Could you check a few things on this model? Use its own coordinates, in mm. A direction names the side the tool comes from. Give positions to 0.01 mm unless a question says otherwise; leave off trailing zeros. Write each loop counter-clockwise with the first axis right and the second up, starting at its lowest first coordinate (ties: lowest second). Pieces come first, ordered by that corner, then holes. Notation, with made-up numbers: M -31.5,73.25 L 7.5,73.25 A28 ccw 7.5,105.25 Z; hole C 5.25,28.5 d10. An arc over 180 degrees is marked long. Use one line per item in the form item = value.
from build123d import *

# Parameters (mm, degrees)
F0_W      = 76.2
F0_H      = 38.1
F1_DEPTH  = 17.78
F2_R      = 6.35
F3_DEPTH  = 15.24
F5_DEPTH  = 5.332479
F6_DEPTH  = 5.837152
F7_R      = 1.27
F8_DEPTH  = 67.31
F9_R      = 5.08
F10_R     = 5.08
F11_W     = 13.054326
F11_H     = 13.088878
F12_DEPTH = 7.62
F13_W     = 11.43
F13_H     = 11.43
F14_DEPTH = 7.62
F15_R     = 2.54
F16_R     = 1.27
F17_DEPTH = 12.7
F18_R     = 2.54


with BuildPart() as f1:
    # F0 (on Front) → F1 (new body)
    with BuildSketch(Plane.XZ):
        Rectangle(F0_W, F0_H)
    extrude(amount=F1_DEPTH)

    # F2 (on face) → F3 (cut)
    with BuildSketch(Plane.XZ.offset(17.78)):
        with Locations((29.285945, 10.045934)):
            Circle(F2_R)
    extrude(amount=-F3_DEPTH, mode=Mode.SUBTRACT)

    # F4 (on face) → F5 (join)
    with BuildSketch(Plane(origin=(-38.1, 0, 0), x_dir=(0, -1, 0), z_dir=(-1, 0, 0))):
        with BuildLine():
            add(Edge.make_bspline(
                [(3.993284, 17.51616), (0.337111, 17.51616), (2.165198, 8.925081), (3.993284, 0.334002), (5.82137, 8.925081), (7.649457, 17.51616), (3.993284, 17.51616)],
                knots=[0, 0, 0, 2.094395, 2.094395, 4.18879, 4.18879, 6.283185, 6.283185, 6.283185], degree=2, weights=[1, 0.5, 1, 0.5, 1, 0.5, 1]))
        make_face()
    extrude(amount=F5_DEPTH)

    # F4 (on face) → F6 (join)
    with BuildSketch(Plane(origin=(-38.1, 0, 0), x_dir=(0, -1, 0), z_dir=(-1, 0, 0))):
        with BuildLine():
            add(Edge.make_bspline(
                [(3.993284, 17.51616), (0.337111, 17.51616), (2.165198, 8.925081), (3.993284, 0.334002), (5.82137, 8.925081), (7.649457, 17.51616), (3.993284, 17.51616)],
                knots=[0, 0, 0, 2.094395, 2.094395, 4.18879, 4.18879, 6.283185, 6.283185, 6.283185], degree=2, weights=[1, 0.5, 1, 0.5, 1, 0.5, 1]))
        make_face()
    extrude(amount=F6_DEPTH)

    # F7 (on face) → F8 (cut)
    with BuildSketch(Plane(origin=(-43.937152, 0, 0), x_dir=(0, -1, 0), z_dir=(-1, 0, 0))):
        with Locations((3.993284, 11.788774)):
            Circle(F7_R)
    extrude(amount=-F8_DEPTH, mode=Mode.SUBTRACT)

    # F9
    f9_edges = [f1.edges().sort_by_distance(p)[0] for p in [
        (38.1, -8.89, 19.05),
    ]]
    fillet(f9_edges, radius=F9_R)

    # F10
    f10_edges = [f1.edges().sort_by_distance(p)[0] for p in [
        (38.1, -8.89, -19.05),
    ]]
    fillet(f10_edges, radius=F10_R)

    # F11 (on face) → F12 (cut)
    with BuildSketch(Plane.XZ.offset(17.78)):
        with Locations((26.983425, -12.505561)):
            Rectangle(F11_W, F11_H)
    extrude(amount=-F12_DEPTH, mode=Mode.SUBTRACT)

    # F13 (on face) → F14 (join)
    with BuildSketch(Plane.XZ.offset(10.16)):
        with Locations((26.983425, -12.505561)):
            Rectangle(F13_W, F13_H)
    extrude(amount=F14_DEPTH)

    # F15
    f15_edges = [f1.edges().sort_by_distance(p)[0] for p in [
        (26.983425, -17.78, -6.790561),
    ]]
    fillet(f15_edges, radius=F15_R)

    # F16 (on face) → F17 (cut)
    with BuildSketch(Plane.XZ.offset(17.78)):
        with Locations((27.043138, -15.251571)):
            Circle(F16_R)
    extrude(amount=-F17_DEPTH, mode=Mode.SUBTRACT)

    # F18
    f18_edges = [f1.edges().sort_by_distance(p)[0] for p in [
        (-38.1, -8.89, -19.05),
    ]]
    fillet(f18_edges, radius=F18_R)


solid = f1.part
1) I want a section at B-B, the plane y = -7. Please give me the cut outline in (x, z).
Checked values:
outline = M -38.1,-16.51 A2.54 ccw -35.56,-19.05 L 33.02,-19.05 A5.08 ccw 38.1,-13.97 L 38.1,13.97 A5.08 ccw 33.02,19.05 L -38.1,19.05 Z; hole C 29.29,10.05 d12.7; hole C 27.04,-15.25 d2.54
2) Thinking about a two-plate mould opening in X: for faces 4 (the flat face through (-1, 0, 0)), 5 (the flat face through (38.1, -9, 0)), 6 (the flat face through (32.698, -14, -13)), which applies, released by +X, released by -X, zero draft, split by the parting line, or undercut?
Checked values:
face_4 = zero draft
face_5 = released by +X
face_6 = undercut
3) For pin 1 Ø3.5 at (x, z) = (27.04, -15.25) entering from +Y; pin 2 Ø4 at (x, y) = (24.5, -15.5) entering from -Z; pin 3 Ø9 at (y, z) = (-8.5, -6.5) entering from -X; pin 4 Ø1.3 at (x, z) = (27.5, -15.5) entering from -Y, each with a flat end and sliding along its axis, tell me the tip position at first contact or that it passes through.
Checked values:
pin_1 = 0
pin_2 = -18.22
pin_3 = -38.1
pin_4 = -5.08
4) For faces 1 (the cylindrical face through (27.1, -17, -7.5)), 2 (the cylindrical face through (-10.753, -5.166, 11.302)), 3 (the flat face through (20.456, -14, -13)), which set-ups out of +Z, -Z, +X, -X, +Y, -Y let a thin tool reach every point of the face, with its end or its side?
Checked values:
face_1 = -Y
face_2 = -X
face_3 = -Z, -Y
5) I want a section at D-D, the plane z = -1. Please give me the cut outline in (x, y).
Checked values:
outline = M -38.1,-17.78 L 38.1,-17.78 L 38.1,0 L -38.1,0 Z
6) I want a section at A-A, the plane z = -11.5. Please give me the cut outline in (x, y).
Checked values:
outline = M -38.1,-17.78 L 20.46,-17.78 L 20.46,-10.16 L 21.27,-10.16 L 21.27,-17.78 L 32.7,-17.78 L 32.7,-10.16 L 33.51,-10.16 L 33.51,-17.78 L 38.1,-17.78 L 38.1,0 L -38.1,0 Z
7) I want a section at C-C, the plane y = -14. Please give me the cut outline in (x, z), plus the area to 3 significant figures.
Checked values:
outline = M -38.1,-16.51 A2.54 ccw -35.56,-19.05 L 20.46,-19.05 L 20.46,-5.96 L 33.51,-5.96 L 33.51,-19.03 A5.08 ccw 38.1,-13.97 L 38.1,13.97 A5.08 ccw 33.02,19.05 L -38.1,19.05 Z; M 21.27,-18.22 L 32.7,-18.22 L 32.7,-6.79 L 21.27,-6.79 Z; hole C 29.29,10.05 d12.7; hole C 27.04,-15.25 d2.54
area = 2,720 mm2
8) If I drill on L1, parallel to X at y = -13.75, z = -10.5; L2, parallel to Z at x = 27.5, y = -10.5; L3, parallel to X at y = -6, z = -5.5, over which ranges is the centre line in solid material (lowest first)?
Checked values:
L1 = -38.1 to 20.46, 21.27 to 32.7, 33.51 to 38.1
L2 = -18.22 to -16.44, -14.07 to -6.79, -5.96 to 3.95, 16.14 to 19.05
L3 = -38.1 to 38.1
